Input: part model. Units: mm. Frame: model coordinates. Face numbers are marked on the shaded views. Round coordinates to 2 decimals unless told otherwise and drop trailing zeros. Write each loop counter-clockwise with the first axis right and the second up, starting at its lowest first coordinate (ties: lowest second). Pieces come first, ordered by that corner, then holes. Notation, with made-up numbers: (56, 56) -> (73, 56) arc R11 cw to (73, 73) -> close; hole circle Ø3 at (24.25, 58.25). An arc over 180 degrees is marked (long way). Write item = value, one per line.
```python
from build123d import *

# Parameters (mm, degrees)
CROQUIS1_R              = 0.75
CROQUIS1_R_2            = 1.5
SALIENTE_EXTRUIR1_DEPTH = 2
CROQUIS2_R              = 4.375
CROQUIS2_R_2            = 2.95
SALIENTE_EXTRUIR2_DEPTH = 3


with BuildPart() as part:
    # Croquis1 → Saliente-Extruir1 (new body)
    with BuildSketch(Plane(origin=(0, 0, 0), x_dir=(1, 0, 0), z_dir=(0, 1, 0))):
        with BuildLine():
            Line((-4, 3.774917218), (-2.382352433, 17.040511421))
            ThreePointArc((-2.382352433, 17.040511421), (0, 19.15), (2.382352433, 17.040511421))
            Line((2.382352433, 17.040511421), (4, 3.774917218))
            ThreePointArc((4, 3.774917218), (0, -5.5), (-4, 3.774917218))
        make_face()
        with Locations(Location((0, 16.75, 0), (0, 0, 270))):
            Circle(CROQUIS1_R, mode=Mode.SUBTRACT)
        with Locations(Location((0, 13.75, 0), (0, 0, 270))):
            Circle(CROQUIS1_R, mode=Mode.SUBTRACT)
        with Locations(Location((0, 10.75, 0), (0, 0, 270))):
            Circle(CROQUIS1_R, mode=Mode.SUBTRACT)
        with Locations(Location((0, 7.75, 0), (0, 0, 270))):
            Circle(CROQUIS1_R, mode=Mode.SUBTRACT)
        with Locations(Location((0, 0, 0), (0, 0, 270))):
            Circle(CROQUIS1_R_2, mode=Mode.SUBTRACT)
    extrude(amount=SALIENTE_EXTRUIR1_DEPTH)

    # Croquis2 → Saliente-Extruir2 (add)
    with BuildSketch(Plane(origin=(0, 2, 0), x_dir=(1, 0, 0), z_dir=(0, 1, 0))):
        with Locations(Location((0, 0, 0), (0, 0, 270))):
            Circle(CROQUIS2_R)
        with Locations(Location((0, 0, 0), (0, 0, 270))):
            Circle(CROQUIS2_R_2, mode=Mode.SUBTRACT)
    extrude(amount=SALIENTE_EXTRUIR2_DEPTH)


solid = part.part
```
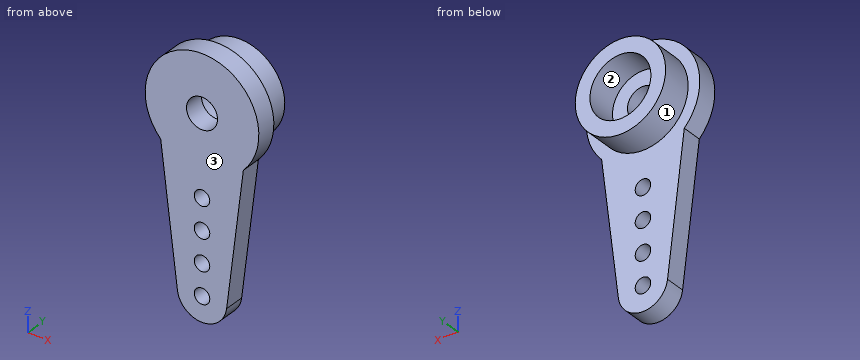
1) Cut plane C-C (y = 1.3). Return the cut outline in (x, z).
Solutions:
outline = (-4, -3.77) -> (-2.38, -17.04) arc R2.4 ccw to (2.38, -17.04) -> (4, -3.77) arc R5.5 ccw (long way) to start; hole circle Ø3 at (0, 0); hole circle Ø1.5 at (0, -16.75); hole circle Ø1.5 at (0, -13.75); hole circle Ø1.5 at (0, -10.75); hole circle Ø1.5 at (0, -7.75)
2) Draft query along Z for the marked faces 1, 2 and 3. Return one class per face: +Z half, -Z half, draft (parallel to the pull), parting line (faces both ways), or undercut.
Solutions:
face_1 = parting line
face_2 = undercut
face_3 = draft
3) Cut plane A-A (z = 0). Return the cut outline in (x, y) (3 decimals).
Solutions:
outline = (-5.5, 0) -> (-1.5, 0) -> (-1.5, 2) -> (-2.95, 2) -> (-2.95, 5) -> (-4.375, 5) -> (-4.375, 2) -> (-5.5, 2) -> close; (1.5, 0) -> (5.5, 0) -> (5.5, 2) -> (4.375, 2) -> (4.375, 5) -> (2.95, 5) -> (2.95, 2) -> (1.5, 2) -> close
4) Line query: L1, parallel to X at y = 0.4, z = 0; L2, parallel to X at y = 2.9, z = 0 (3 decimals); L3, parallel to Y at x = -4.5, z = -0.5. Output: solid intervals per line, ascending. Write a range as from..to.
Solutions:
L1 = -5.5..-1.5, 1.5..5.5
L2 = -4.375..-2.95, 2.95..4.375
L3 = 0..2
5) Cut plane B-B (x = 1.25). Return the cut outline in (y, z).
Solutions:
outline = (0, -18.8) -> (2, -18.8) -> (2, -4.19) -> (5, -4.19) -> (5, -2.67) -> (2, -2.67) -> (2, -0.83) -> (0, -0.83) -> close; (0, 0.83) -> (2, 0.83) -> (2, 2.67) -> (5, 2.67) -> (5, 4.19) -> (2, 4.19) -> (2, 5.36) -> (0, 5.36) -> close
6) Cut plane D-D (z = -13.75). Return the cut outline in (x, y).
Solutions:
outline = (-2.78, 0) -> (-0.75, 0) -> (-0.75, 2) -> (-2.78, 2) -> close; (0.75, 0) -> (2.78, 0) -> (2.78, 2) -> (0.75, 2) -> close
7) First-contact query: P1, Ø0.9, axis at x = 0, z = -10.75, coming from the -Y side; P2, Ø3.5, axis at x = 0, z = 0, coming from the +Y side; P3, Ø1.7, axis at x = 0, z = -13.75, coming from the -Y side; P4, Ø1, axis at x = 3.5, y = 2, coming from the +Z side. Flat tips, straight axial feed; report the tip coordinate or a pass-through.
Solutions:
P1 = through
P2 = 2
P3 = 0
P4 = 4.61
